from build123d import *

# Parameters (mm, degrees)
F0_R     = 25.4
F0_R_2   = 7
F1_DEPTH = 3.175


with BuildPart() as f1:
    # F0 (on Top) → F1 (new body)
    with BuildSketch(Plane.XY):
        Circle(F0_R)
        with BuildLine():
            Line((-0.518496, -13.15886), (0.497504, -13.15886))
            ThreePointArc((0.497504, -13.15886), (1.39553, -13.530834), (1.767504, -14.42886))
            Line((1.767504, -14.42886), (1.767504, -18.23886))
            ThreePointArc((1.767504, -18.23886), (1.39553, -19.136886), (0.497504, -19.50886))
            Line((0.497504, -19.50886), (-0.518496, -19.50886))
            ThreePointArc((-0.518496, -19.50886), (-1.416522, -19.136886), (-1.788496, -18.23886))
            Line((-1.788496, -18.23886), (-1.788496, -14.42886))
            ThreePointArc((-1.788496, -14.42886), (-1.416522, -13.530834), (-0.518496, -13.15886))
        make_face(mode=Mode.SUBTRACT)
        Circle(F0_R_2, mode=Mode.SUBTRACT)
        with BuildLine():
            Line((-0.508, 19.375), (0.508, 19.375))
            ThreePointArc((0.508, 19.375), (1.406026, 19.003026), (1.778, 18.105))
            Line((1.778, 18.105), (1.778, 14.295))
            ThreePointArc((1.778, 14.295), (1.406026, 13.396974), (0.508, 13.025))
            Line((0.508, 13.025), (-0.508, 13.025))
            ThreePointArc((-0.508, 13.025), (-1.406026, 13.396974), (-1.778, 14.295))
            Line((-1.778, 14.295), (-1.778, 18.105))
            ThreePointArc((-1.778, 18.105), (-1.406026, 19.003026), (-0.508, 19.375))
        make_face(mode=Mode.SUBTRACT)
    extrude(amount=F1_DEPTH)


solid = f1.part
Design review of the part built by this model. Coordinates are the model's own, in mm. A direction names the side the tool comes from. Round coordinates to 2 decimals unless told otherwise and drop trailing zeros. Write each loop counter-clockwise with the first axis right and the second up, starting at its lowest first coordinate (ties: lowest second). Pieces come first, ordered by that corner, then holes. Notation, with made-up numbers: (8.5, 75) -> (67.5, 75) arc R25 cw to (67.5, 112) -> close; hole circle Ø10 at (44.25, 69). An arc over 180 degrees is marked (long way). One line per item, written item: value. Start each with the question number.
Q1. The part is to be moulded in two halves that separate along Y. For faces 1 (the face through (1.386, -13.521, 1.565)), 2 (the face through (-5.506, -24.796, 1.565)), 3 (the face through (5.3, -5.3, 0)), say which applies: pulls with the +Y half, pulls with the -Y half, needs draft (parallel to the pull), parting line crosses it, or undercut.
Q2. Tool access review of faces 4 (the face through (5.3, -5.3, 3.175)), 5 (the face through (-1.788, -16, 2)): name each direction out of +Z, -Z, +X, -X, +Y, -Y from which nothing blocks a thin tool from reaching the whole face with its end or side.
Q3. To check wall thickness, follow probe 1 along Y at (x, z) = (0, 0.95) (3 decimals); probe 2 along X at (y, z) = (17.5, 1.55); probe 3 along X at (y, z) = (4, 1.55). State the ranges of each line that lie inside material, in increasing order.
Q4. Add section B-B (z = 0.95). Give the boundary of the cut face in (x, y) (1 decimal), then the cut area to 3 significant figures.
Q5. Add section D-D (y = -11.5). Give the boundary of the cut face in (x, z) (3 decimals), then the cut area to 3 significant figures.
Q6. Add section A-A (y = 0). Give the boundary of the cut face in (x, z) (3 decimals), then the cut area to 3 significant figures.
Q7. Add section C-C (x = -11). Give the boundary of the cut face in (y, z) (3 decimals).
Q8. Insertion check: P1, Ø1.6, axis at y = 15.5, z = 2, coming from the -X side; P2, Ø8.5, axis at x = 0, y = 0, coming from the -Z side; P3, Ø1.1, axis at x = 0, z = 1, coming from the -Y side; P4, Ø1.1, axis at x = 0, z = 1, coming from the +Y side. Each pin has a flat end and moves straight along its axis. Give the tip position at first contact, or say it passes through.
Response:
1. face 1: undercut
1. face 2: parting line crosses it
1. face 3: needs draft
2. face 4: +Z, +X, -X, +Y, -Y
2. face 5: +Z, -Z
3. probe 1: y = -25.4 to -19.509, -13.159 to -7, 7 to 13.025, 19.375 to 25.4
3. probe 2: x = -18.41 to -1.78, 1.78 to 18.41
3. probe 3: x = -25.08 to -5.74, 5.74 to 25.08
4. outline: circle Ø50.8 at (0, 0); hole circle Ø14 at (0, 0); hole (-1.8, -18.2) arc R1.3 ccw to (-0.5, -19.5) -> (0.5, -19.5) arc R1.3 ccw to (1.8, -18.2) -> (1.8, -14.4) arc R1.3 ccw to (0.5, -13.2) -> (-0.5, -13.2) arc R1.3 ccw to (-1.8, -14.4) -> close; hole (-1.8, 14.3) arc R1.3 ccw to (-0.5, 13) -> (0.5, 13) arc R1.3 ccw to (1.8, 14.3) -> (1.8, 18.1) arc R1.3 ccw to (0.5, 19.4) -> (-0.5, 19.4) arc R1.3 ccw to (-1.8, 18.1) -> close
4. area: 1,830 mm^2
5. outline: (-22.648, 0) -> (22.648, 0) -> (22.648, 3.175) -> (-22.648, 3.175) -> close
5. area: 144 mm^2
6. outline: (-25.4, 0) -> (-7, 0) -> (-7, 3.175) -> (-25.4, 3.175) -> close; (7, 0) -> (25.4, 0) -> (25.4, 3.175) -> (7, 3.175) -> close
6. area: 117 mm^2
7. outline: (-22.895, 0) -> (22.895, 0) -> (22.895, 3.175) -> (-22.895, 3.175) -> close
8. P1: stops at x = -20.71
8. P2: passes through
8. P3: stops at y = -25.4
8. P4: stops at y = 25.4
